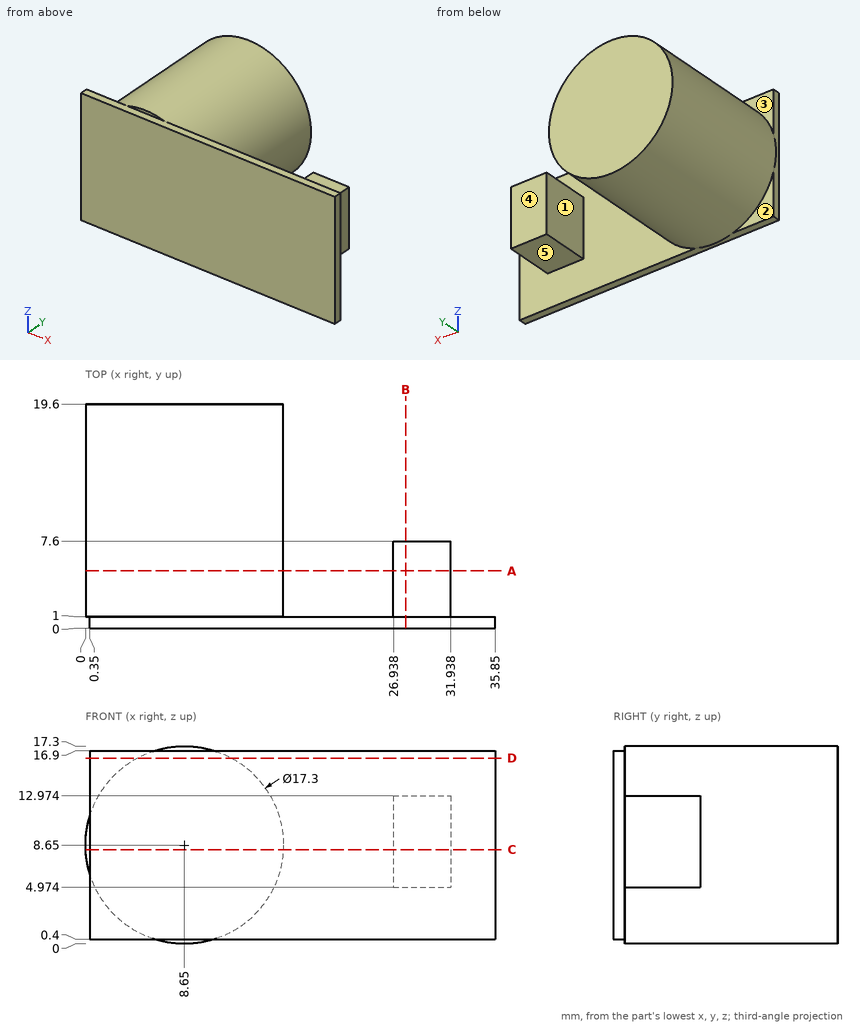
Study the drawing (mm; zero at the part's minimum x, y, z) and answer. A direction names the side the tool comes from. Coordinates: 2 decimals unless noted, no trailing zeros. Write each loop counter-clockwise with the first axis right and the second up, starting at its lowest first coordinate (ties: lowest second). Pieces come first, ordered by that corner, then holes. Notation, with made-up numbers: (57, 22) -> (103, 22) arc R16 cw to (103, 30) -> close; hole circle Ø4 at (-10.5, 23.5). An arc over 180 degrees is marked (long way). Write item = value, one per line.
(1) Section A-A on y = 5 is taken. Write down the section's boundary in (x, z), plus the area to 3 significant figures.
From the geometry:
outline = circle Ø17.3 at (8.65, 8.65); (26.94, 4.97) -> (31.94, 4.97) -> (31.94, 12.97) -> (26.94, 12.97) -> close
area = 275 mm2
(2) Section B-B on x = 28 is taken. Write down the section's boundary in (y, z), plus the area to 3 significant figures.
From the geometry:
outline = (0, 0.4) -> (1, 0.4) -> (1, 4.97) -> (7.6, 4.97) -> (7.6, 12.97) -> (1, 12.97) -> (1, 16.9) -> (0, 16.9) -> close
area = 69.3 mm2
(3) Which of the six approach directions +Z, -Z, +X, -X, +Y, -Y give full straight-line access (tool end or side, diameter ignored) to the marked faces 3, 4 and 5?
From the geometry:
face_3 = +Z, -X, +Y
face_4 = +Z, -Z, +X, +Y
face_5 = -Z, +X, +Y
(4) Section D-D on z = 16.25 is taken. Write down the section's boundary in (x, y).
From the geometry:
outline = (0.35, 0) -> (35.85, 0) -> (35.85, 1) -> (12.78, 1) -> (12.78, 19.6) -> (4.52, 19.6) -> (4.52, 1) -> (0.35, 1) -> close
(5) For a pull along X with two mould halves and no side action, classify the marked faces 1 and 2 as +X half, -X half, draft (parallel to the pull), parting line (faces both ways), or undercut.
From the geometry:
face_1 = undercut
face_2 = draft
(6) Straight lines are drawn through the part: L1, parallel to Y at x = 24, z = 7; L2, parallel to Z at x = 30, y = 3; L3, parallel to Y at x = 30, z = 11. For each, find the intervals that lie inside material, in ascending order. Write a range as from..to.
From the geometry:
L1 = 0..1
L2 = 4.97..12.97
L3 = 0..7.6
(7) Given pin 1 Ø8 at (y, z) = (2, 13) entering from -X; pin 2 Ø1.5 at (x, y) = (29, 5) entering from -Z; pin 3 Ø4 at (y, z) = (16, 12.5) entering from +X, each flat-ended and moving along its own axis, determine where each tip first touches the part or whether it passes through.
From the geometry:
pin_1 = 0.01
pin_2 = 4.97
pin_3 = 17.1
(8) Section C-C on z = 8.25 is taken. Write down the section's boundary in (x, y), plus the area to 3 significant figures.
From the geometry:
outline = (0.01, 1) -> (0.35, 1) -> (0.35, 0) -> (35.85, 0) -> (35.85, 1) -> (31.94, 1) -> (31.94, 7.6) -> (26.94, 7.6) -> (26.94, 1) -> (17.29, 1) -> (17.29, 19.6) -> (0.01, 19.6) -> close
area = 390 mm2
